The figure shows three views and two pictorial views of one solid part (mm, origin at its lowest corner). Answer the questions. Give positions to 0.01 mm unless a question says otherwise; leave off trailing zeros. Order: outer loops, then holes, each group sorted by start corner. A loop starts at its lowest first (then second) coordinate and runs counter-clockwise, first axis right, second up. Notation, with made-up numbers: (25, -10) - (33, -10) arc R34 cw to (33, 21) - close; hole circle Ø5 at (39.25, 33.5). An arc over 180 degrees is marked (long way). Answer as CSV lines item,"result". Start each with the question number.
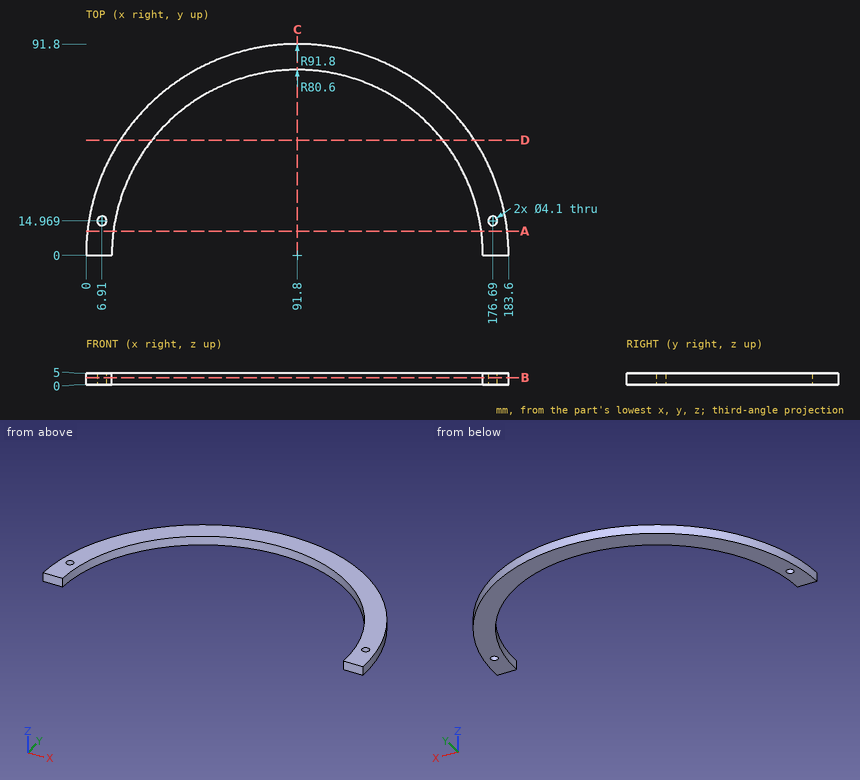
(1) Section C-C, the plane x = 91.8 is taken. Write down the section's boundary in (y, z).
(2) Section B-B, the plane z = 3.15 is taken. Write down the section's boundary in (x, y).
(3) Flat-ended cylindrical pins translate along their axes: pin 1 Ø5 at (x, y) = (25.5, 36.5) entering from -Z; pin 2 Ø5.5 at (x, y) = (6.91, 14.97) entering from +Z. Find the tip coordinate at first contact, or state that the pin passes through.
(4) Section A-A, the plane y = 10.5 is taken. Write down the section's boundary in (x, z).
(5) Straight lines are drawn through the part: line 1 (X direction, y = 15, z = 3.8) (1 decimal); line 2 (X direction, y = 63.5, z = 2.2) (1 decimal); line 3 (X direction, y = 68.5, z = 3) (1 decimal). For each, find the intervals that lie inside material, in ascending order. Write a range as [from, to].
(6) Section D-D, the plane y = 50 is taken. Write down the section's boundary in (x, z).
Checks:
1,outline,"(80.6, 0) - (91.8, 0) - (91.8, 5) - (80.6, 5) - close"
2,outline,"(0, 0) - (11.2, 0) arc R80.6 cw to (172.4, 0) - (183.6, 0) arc R91.8 ccw to start; hole circle Ø4.1 at (6.91, 14.97); hole circle Ø4.1 at (176.69, 14.97)"
3,pin 1,"passes through"
3,pin 2,"stops at z = 5"
4,outline,"(0.6, 0) - (11.89, 0) - (11.89, 5) - (0.6, 5) - close; (171.71, 0) - (183, 0) - (183, 5) - (171.71, 5) - close"
5,line 1,"x = [1.2, 4.9], [9, 12.6], [171, 174.6], [178.7, 182.4]"
5,line 2,"x = [25.5, 42.2], [141.4, 158.1]"
5,line 3,"x = [30.7, 49.3], [134.3, 152.9]"
6,outline,"(14.81, 0) - (28.58, 0) - (28.58, 5) - (14.81, 5) - close; (155.02, 0) - (168.79, 0) - (168.79, 5) - (155.02, 5) - close"
